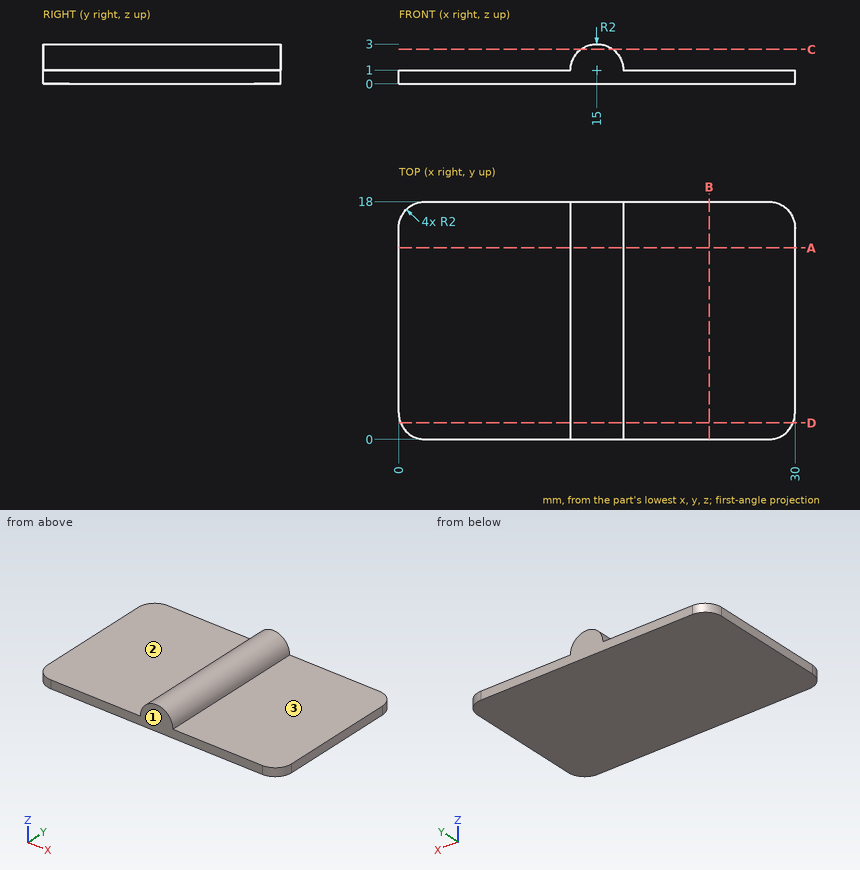
Job drawing, mm, ordinate dimensions from the low corner. One solid piece. A direction names the side the tool comes from. Round coordinates to 2 decimals unless told otherwise and drop trailing zeros. Order: outer loops, then holes, each group sorted by start corner. A loop starts at its lowest first (then second) coordinate and runs counter-clockwise, first axis right, second up. Notation, with made-up numbers: (52, 75) -> (90, 75) arc R25 cw to (90, 105) -> close; hole circle Ø8 at (51.5, 2). An arc over 180 degrees is marked (long way). Answer in a Markdown table with one row per item.
1) Band-saw the part on C-C on z = 2.6. Give the cut face in (x, y).
Values:
| item | result |
|---|---|
| outline | (13.8, 0) -> (16.2, 0) -> (16.2, 18) -> (13.8, 18) -> close |
2) Which spindle directions (+Z, -Z, +X, -X, +Y, -Y) get a long thin tool onto all of the face, cutting with end or side? Do the marked faces 1, 2 and 3. Say none if no direction does.
Values:
| item | result |
|---|---|
| face 1 | +Z, -Z, +X, -X, -Y |
| face 2 | +Z, -X, +Y, -Y |
| face 3 | +Z, +X, +Y, -Y |
3) Band-saw the part on D-D on y = 1.25. Give the cut face in (x, z), and give its area (3 significant figures).
Values:
| item | result |
|---|---|
| outline | (0.15, 0) -> (29.85, 0) -> (29.85, 1) -> (17, 1) arc R2 ccw to (13, 1) -> (0.15, 1) -> close |
| area | 36.0 mm2 |
4) Wall check: L1, parallel to Z at x = 18, y = 4.25; L2, parallel to X at y = 7.25, z = 1.1; L3, parallel to X at y = 13, z = 2.3. Give the ranges that are in metal, low to high.
Values:
| item | result |
|---|---|
| L1 | 0 to 1 |
| L2 | 13 to 17 |
| L3 | 13.48 to 16.52 |
5) Pin check, flat tips, straight feed: P1, Ø1, axis at y = 11.5, z = 2, coming from the +X side; P2, Ø1, axis at y = 11.5, z = 2.5, coming from the -X side; P3, Ø1.5, axis at y = 8.5, z = 2.5, coming from the -X side. Stop position of each tip, or through.
Values:
| item | result |
|---|---|
| P1 | x = 16.94 |
| P2 | x = 13.27 |
| P3 | x = 13.15 |
6) Band-saw the part on A-A on y = 14.5. Give the cut face in (x, z), and give its area (3 significant figures).
Values:
| item | result |
|---|---|
| outline | (0, 0) -> (30, 0) -> (30, 1) -> (17, 1) arc R2 ccw to (13, 1) -> (0, 1) -> close |
| area | 36.3 mm2 |
7) Band-saw the part on B-B on x = 23.5. Give the cut face in (y, z), and give its area (3 significant figures).
Values:
| item | result |
|---|---|
| outline | (0, 0) -> (18, 0) -> (18, 1) -> (0, 1) -> close |
| area | 18.0 mm2 |
